Geometry: final body of the model. Coordinates: model frame, mm. Face numbers are marked on the shaded views. A direction names the side the tool comes from. Round coordinates to 2 decimals unless told otherwise and drop trailing zeros. Loops run counter-clockwise (first coordinate to the right, second up) from the corner with the lowest first, then second, coordinate; pieces in that order, holes last. Notation, with made-up numbers: (-24, 79.25) -> (-8, 79.25) arc R17 ccw to (-8, 106.25) -> close; hole circle Ø5 at (71, 80.25). An arc over 180 degrees is marked (long way). Answer in a Markdown table with one row per item.
```python
from build123d import *

# Parameters (mm, degrees)
SALIENTE_EXTRUIR1_DEPTH = 60


with BuildPart() as part:
    # Croquis1 → Saliente-Extruir1 (new body)
    with BuildSketch(Plane.XY):
        with BuildLine():
            Line((-8.57523763, 59.384049202), (-10, 30))
            Line((-10, 30), (10, 30))
            Line((10, 30), (10, 59.160797831))
            ThreePointArc((10, 59.160797831), (43.028053102, 41.816105106), (59.422289674, 8.306111602))
            Line((59.422289674, 8.306111602), (30, 8.306111602))
            Line((30, 8.306111602), (30, -8.306111602))
            Line((30, -8.306111602), (59.422289674, -8.306111602))
            ThreePointArc((59.422289674, -8.306111602), (43.028053102, -41.816105106), (10, -59.160797831))
            Line((10, -59.160797831), (10, -30))
            Line((10, -30), (-10, -30))
            Line((-10, -30), (-8.57523763, -59.384049202))
            ThreePointArc((-8.57523763, -59.384049202), (-42.52240418, -42.330191858), (-59.422289674, -8.306111602))
            Line((-59.422289674, -8.306111602), (-30, -8.306111602))
            Line((-30, -8.306111602), (-30, 8.306111602))
            Line((-30, 8.306111602), (-59.422289674, 8.306111602))
            ThreePointArc((-59.422289674, 8.306111602), (-42.52240418, 42.330191858), (-8.57523763, 59.384049202))
        make_face()
    extrude(amount=SALIENTE_EXTRUIR1_DEPTH)


solid = part.part
```
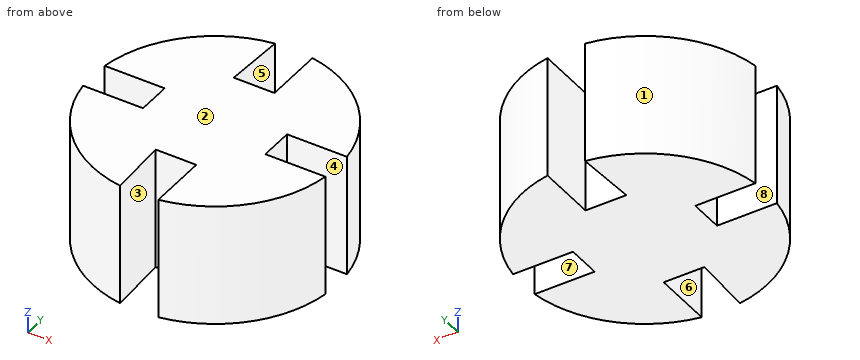
Item 1: First-contact query: P1, Ø4, axis at y = -37.5, z = 31.5, coming from the +X side; P2, Ø10, axis at x = 4, z = 43.5, coming from the -Y side; P3, Ø6, axis at x = -32, z = 50.5, coming from the +Y side. Flat tips, straight axial feed; report the tip coordinate or a pass-through.
Ans:
| item | result |
|---|---|
| P1 | x = 48.37 |
| P2 | y = -30 |
| P3 | y = 52.53 |
Item 2: Set-up query: the marked faces 5, 6, 7 and 8. Return all of +Z, -Z, +X, -X, +Y, -Y with unobstructed straight access to the full face (end or side cutting, diameter ignored); none if empty.
Ans:
| item | result |
|---|---|
| face 5 | +Z, -Z |
| face 6 | +Z, -Z, -Y |
| face 7 | +Z, -Z, +X |
| face 8 | +Z, -Z, -X |
Item 3: Section query B-B, the plane x = 41.5. Output: boundary loops of the cut face in (y, z), and give its area (3 significant figures).
Ans:
| item | result |
|---|---|
| outline | (-43.33, 0) -> (-8.31, 0) -> (-8.31, 60) -> (-43.33, 60) -> close; (8.31, 0) -> (43.33, 0) -> (43.33, 60) -> (8.31, 60) -> close |
| area | 4,200 mm2 |
Item 4: Ray query, L1, parallel to X at y = -8, z = 50; L2, parallel to X at y = 43, z = 44; L3, parallel to X at y = 48.5, z = 18. Return the intervals inside material, ascending.
Ans:
| item | result |
|---|---|
| L1 | -30 to 30 |
| L2 | -41.84 to -9.37, 10 to 41.84 |
| L3 | -35.32 to -9.1, 10 to 35.32 |
Item 5: Section query D-D, the plane y = 5.5. Output: boundary loops of the cut face in (x, z).
Ans:
| item | result |
|---|---|
| outline | (-30, 0) -> (30, 0) -> (30, 60) -> (-30, 60) -> close |
Item 6: Section query A-A, the plane y = -51. Output: boundary loops of the cut face in (x, z).
Ans:
| item | result |
|---|---|
| outline | (-31.61, 0) -> (-8.98, 0) -> (-8.98, 60) -> (-31.61, 60) -> close; (10, 0) -> (31.61, 0) -> (31.61, 60) -> (10, 60) -> close |
Item 7: Mould query, pull axis Y, two halves, no side actions, for the marked faces 1, 2, 3 and 4. Classes: released by +Y, released by -Y, zero draft, split by the parting line, or undercut.
Ans:
| item | result |
|---|---|
| face 1 | released by +Y |
| face 2 | zero draft |
| face 3 | undercut |
| face 4 | undercut |
Item 8: Section query C-C, the plane z = 40.5. Output: boundary loops of the cut face in (x, y).
Ans:
| item | result |
|---|---|
| outline | (-59.42, -8.31) arc R60 ccw to (-8.58, -59.38) -> (-10, -30) -> (10, -30) -> (10, -59.16) arc R60 ccw to (59.42, -8.31) -> (30, -8.31) -> (30, 8.31) -> (59.42, 8.31) arc R60 ccw to (10, 59.16) -> (10, 30) -> (-10, 30) -> (-8.58, 59.38) arc R60 ccw to (-59.42, 8.31) -> (-30, 8.31) -> (-30, -8.31) -> close |
